```python
from build123d import *

# Parameters (mm, degrees)
CSK_FOR_M2_COUNTERSUNK_FLAT_HEAD_SCREW1_D           = 2.2
CSK_FOR_M2_COUNTERSUNK_FLAT_HEAD_SCREW1_CSINK_D     = 4.4
CSK_FOR_M2_COUNTERSUNK_FLAT_HEAD_SCREW1_CSINK_ANGLE = 90
CUT_EXTRUDE1_DEPTH                                  = 9.319
CUT_EXTRUDE1_DEPTH_BACK                             = 1.3
FILLET1_R                                           = 3
FILLET2_R                                           = 2
CUT_EXTRUDE3_START                                  = -1.35
CUT_EXTRUDE3_DEPTH                                  = 1.35
M4_TAPPED_HOLE2_D                                   = 3.3
M4_TAPPED_HOLE2_DEPTH                               = 10.1
M4_TAPPED_HOLE2_TIP                                 = 0.991420021
M2_5_TAPPED_HOLE1_D                                 = 2.05
M2_5_TAPPED_HOLE1_DEPTH                             = 6.35
M2_5_TAPPED_HOLE1_TIP                               = 0.615882135
CUT_EXTRUDE4_REACH                                  = 51.335
SKETCH11_OUTSIDE_W                                  = 62.978
SKETCH11_OUTSIDE_H                                  = 62.978
CUT_EXTRUDE2_DEPTH                                  = 50.335229157
FILLET3_R                                           = 1
CHAMFER1_SIZE                                       = 1
M4_TAPPED_HOLE1_AT_2_COUNT                          = 2
M4_TAPPED_HOLE1_AT_2_PITCH                          = 22
FILLET4_R                                           = 0.5


with BuildPart() as part:
    # Sketch1 → Revolve1 (revolve)
    with BuildSketch(Plane(origin=(0, 0, 0), x_dir=(0, 0, -1), z_dir=(1, 0, 0))):
        Polygon((13.2, 3.5), (13.2, 18.844), (15, 18.844), (15, 37.094), (23, 37.094), (23, 16.013248777), (23, 0), (8.5, 0), (5.5, 0), (5.5, 1.35), (3.75, 1.35), (3.75, 3.5), align=None)
    revolve(axis=Axis((0, 0, 0), (0, 1, 0)))

    # CSK for M2 Countersunk Flat Head Screw1 (through all)
    with Locations(Plane(origin=(0, 3.5, 0), x_dir=(1, 0, 0), z_dir=(0, 1, 0))):
        with Locations((0, 6.5), (-5.629165125, -3.25), (5.629165125, -3.25)):
            CounterSinkHole(CSK_FOR_M2_COUNTERSUNK_FLAT_HEAD_SCREW1_D / 2, CSK_FOR_M2_COUNTERSUNK_FLAT_HEAD_SCREW1_CSINK_D / 2, counter_sink_angle=CSK_FOR_M2_COUNTERSUNK_FLAT_HEAD_SCREW1_CSINK_ANGLE)

    # Sketch5 → Cut-Extrude1 (cut, two sides: drawn at the far end of the back side and taken through both)
    with BuildSketch(Plane(origin=(0, 3.5, 0), x_dir=(1, 0, 0), z_dir=(0, 1, 0)).offset(-CUT_EXTRUDE1_DEPTH_BACK)):
        with BuildLine():
            Line((-13.5, -18.62122445), (-13.5, -29.562959847))
            Line((-13.5, -29.562959847), (13.5, -29.562959847))
            Line((13.5, -29.562959847), (13.5, -18.62122445))
            ThreePointArc((13.5, -18.62122445), (16.584015432, -15.936449797), (19.14388926, -12.748))
            Line((19.14388926, -12.748), (13.93421226, -12.748))
            Line((13.93421226, -12.748), (7.5, -6.748))
            Line((7.5, -6.748), (-7.5, -6.748))
            Line((-7.5, -6.748), (-13.93421226, -12.748))
            Line((-13.93421226, -12.748), (-19.14388926, -12.748))
            ThreePointArc((-19.14388926, -12.748), (-16.584015432, -15.936449797), (-13.5, -18.62122445))
        make_face()
    extrude(amount=CUT_EXTRUDE1_DEPTH + CUT_EXTRUDE1_DEPTH_BACK, mode=Mode.SUBTRACT)

    # Fillet1
    fillet1_edges = [part.edges().sort_by_distance(p)[0] for p in [
        (-19.14388926, 7.5095, 12.748),
        (-13.93421226, 7.5095, 12.748),
        (13.93421226, 7.5095, 12.748),
        (19.14388926, 7.5095, 12.748),
    ]]
    fillet(fillet1_edges, radius=FILLET1_R)

    # Fillet2
    fillet2_edges = [part.edges().sort_by_distance(p)[0] for p in [
        (12.06906123, 3.5, -5.345817152),
    ]]
    fillet(fillet2_edges, radius=FILLET2_R)

    # Sketch14 → Cut-Extrude3 (cut)
    with BuildSketch(Plane.XZ.offset(CUT_EXTRUDE3_START)):
        with BuildLine():
            Line((1.1, -6.5), (1.1, -5.388877434))
            ThreePointArc((1.1, -5.388877434), (4.763139721, -2.75), (5.216904756, 1.741810773))
            Line((5.216904756, 1.741810773), (6.179165125, 2.297372056))
            ThreePointArc((6.179165125, 2.297372056), (6.581793069, 3.8), (5.079165125, 4.202627944))
            Line((5.079165125, 4.202627944), (4.116904756, 3.647066661))
            ThreePointArc((4.116904756, 3.647066661), (0, 5.5), (-4.116904756, 3.647066661))
            Line((-4.116904756, 3.647066661), (-5.079165125, 4.202627944))
            ThreePointArc((-5.079165125, 4.202627944), (-6.581793069, 3.8), (-6.179165125, 2.297372056))
            Line((-6.179165125, 2.297372056), (-5.216904756, 1.741810773))
            ThreePointArc((-5.216904756, 1.741810773), (-4.763139721, -2.75), (-1.1, -5.388877434))
            Line((-1.1, -5.388877434), (-1.1, -6.5))
            ThreePointArc((-1.1, -6.5), (0, -7.6), (1.1, -6.5))
        make_face()
    extrude(amount=CUT_EXTRUDE3_DEPTH, mode=Mode.SUBTRACT)

    # M4 Tapped Hole2
    with Locations(Plane(origin=(0, 37.094, 0), x_dir=(-1, 0, 0), z_dir=(0, 1, 0))):
        with Locations((16.454482672, 9.5), (0, -19), (-16.454482672, 9.5)):
            Hole(M4_TAPPED_HOLE2_D / 2, depth=M4_TAPPED_HOLE2_DEPTH)
            with Locations((0, 0, -(M4_TAPPED_HOLE2_DEPTH + M4_TAPPED_HOLE2_TIP / 2))):  # 118° drill point
                Cone(0, M4_TAPPED_HOLE2_D / 2, M4_TAPPED_HOLE2_TIP, mode=Mode.SUBTRACT)

    # M2.5 Tapped Hole1
    with Locations(Plane(origin=(0, 12.819, 0), x_dir=(-1, 0, 0), z_dir=(0, -1, 0))):
        with Locations((-10.4775, -15.748), (10.4775, -15.748)):
            Hole(M2_5_TAPPED_HOLE1_D / 2, depth=M2_5_TAPPED_HOLE1_DEPTH)
            with Locations((0, 0, -(M2_5_TAPPED_HOLE1_DEPTH + M2_5_TAPPED_HOLE1_TIP / 2))):  # 118° drill point
                Cone(0, M2_5_TAPPED_HOLE1_D / 2, M2_5_TAPPED_HOLE1_TIP, mode=Mode.SUBTRACT)

    # Sketch15 → Cut-Extrude4 (cut, up to next)
    with BuildSketch(Plane.XZ, mode=Mode.PRIVATE) as cut_extrude4_sk1:
        with BuildLine():
            Line((15.115943687, 12.748), (17.463576266, 12.748))
            ThreePointArc((17.463576266, 12.748), (18.982358673, 12.335141279), (20.083112706, 11.2102))
            ThreePointArc((20.083112706, 11.2102), (0, 23), (-20.083112706, 11.2102))
            ThreePointArc((-20.083112706, 11.2102), (-18.982358673, 12.335141279), (-17.463576266, 12.748))
            Line((-17.463576266, 12.748), (-15.115943687, 12.748))
            Line((-15.115943687, 12.748), (15.115943687, 12.748))
        make_face()
    cut_extrude4_tool1 = extrude(cut_extrude4_sk1.sketch, amount=-CUT_EXTRUDE4_REACH, mode=Mode.PRIVATE) & part.part
    add(cut_extrude4_tool1.solids().sort_by_distance((0, 0, 16.923735))[0], mode=Mode.SUBTRACT)

    # Sketch11 outside → Cut-Extrude2 (cut, through all)
    with BuildSketch(Plane(origin=(0, 0, 0), x_dir=(1, 0, 0), z_dir=(0, 1, 0))):
        Rectangle(SKETCH11_OUTSIDE_W, SKETCH11_OUTSIDE_H)
        with BuildLine():
            Line((13.983717047, 18.260768263), (20.411593144, 10.600323832))
            ThreePointArc((20.411593144, 10.600323832), (0, -23), (-20.411593144, 10.600323832))
            Line((-20.411593144, 10.600323832), (-13.983717047, 18.260768263))
            ThreePointArc((-13.983717047, 18.260768263), (0, 23), (13.983717047, 18.260768263))
        make_face(mode=Mode.SUBTRACT)
    extrude(amount=CUT_EXTRUDE2_DEPTH, mode=Mode.SUBTRACT)

    # Fillet3
    # the kernel refuses this fillet: 1 mm, written as the material it takes off along each edge
    with BuildSketch(Plane(origin=(0, 0, 0), x_dir=(-0.8322161318186808, 0, -0.5544513594002202), z_dir=(0.5544513594002202, 0, -0.8322161318186808))) as fillet3_piece_1:
        with BuildLine():
            CenterArc((23 - FILLET3_R, FILLET3_R), FILLET3_R, 270, 90)
            Line((23 - FILLET3_R, 0), (23, 0))
            Line((23, 0), (23, FILLET3_R))
        make_face()
    revolve(axis=Axis((0, 0, 0), (0, 1, 0)), revolution_arc=62.84276799, mode=Mode.SUBTRACT)
    with BuildSketch(Plane(origin=(17.463576266, 0, 9.748), x_dir=(0, 0, 1), z_dir=(-1, 0, 0))) as fillet3_piece_2:
        with BuildLine():
            CenterArc((3 - FILLET3_R, FILLET3_R), FILLET3_R, 270, 90)
            Line((3, FILLET3_R), (3, 0))
            Line((3, 0), (3 - FILLET3_R, 0))
        make_face()
    revolve(axis=Axis((17.463576266, 0, 9.748), (0, 1, 0)), revolution_arc=60.830166101, mode=Mode.SUBTRACT)
    with BuildSketch(Plane(origin=(-17.463576266, 0, 9.748), x_dir=(-0.8731788133022929, 0, 0.48739999999999956), z_dir=(-0.48739999999999956, 0, -0.8731788133022929))) as fillet3_piece_3:
        with BuildLine():
            CenterArc((3 - FILLET3_R, FILLET3_R), FILLET3_R, 270, 90)
            Line((3 - FILLET3_R, 0), (3, 0))
            Line((3, 0), (3, FILLET3_R))
        make_face()
    revolve(axis=Axis((-17.463576266, 0, 9.748), (0, 1, 0)), revolution_arc=60.830166101, mode=Mode.SUBTRACT)
    with BuildSketch(Plane(origin=(17.463576266, 0, 12.748), x_dir=(0, 1, 0), z_dir=(-1, 0, 0))) as fillet3_piece_4:
        with BuildLine():
            CenterArc((FILLET3_R, FILLET3_R), FILLET3_R, 180, 90)
            Line((0, FILLET3_R), (0, 0))
            Line((0, 0), (FILLET3_R, 0))
        make_face()
    extrude(amount=34.927152532, mode=Mode.SUBTRACT)
    with BuildSketch(Plane(origin=(0, 37.094, 0), x_dir=(-0.8320605059369173, 0, -0.5546848785211302), z_dir=(0.5546848785211302, 0, -0.8320605059369173))) as fillet3_piece_5:
        with BuildLine():
            CenterArc((23 - FILLET3_R, -FILLET3_R), FILLET3_R, 0, 90)
            Line((23 - FILLET3_R, 0), (23, 0))
            Line((23, 0), (23, -FILLET3_R))
        make_face()
    revolve(axis=Axis((0, 37.094, 0), (0, 1, 0)), revolution_arc=247.378025481, mode=Mode.SUBTRACT)
    with BuildSketch(Plane(origin=(0, 37.094, 0), x_dir=(0.6905501820120585, 0, -0.7232844849180111), z_dir=(0.7232844849180111, 0, 0.6905501820120585))) as fillet3_piece_6:
        with BuildLine():
            CenterArc((23 - FILLET3_R, -FILLET3_R), FILLET3_R, 0, 90)
            Line((23 - FILLET3_R, 0), (23, 0))
            Line((23, 0), (23, -FILLET3_R))
        make_face()
    revolve(axis=Axis((0, 37.094, 0), (0, 1, 0)), revolution_arc=87.347352667, mode=Mode.SUBTRACT)
    with BuildSketch(Plane(origin=(0, 0, 0), x_dir=(-0.6905501820120575, 0, -0.7232844849180122), z_dir=(-0.7232844849180122, 0, 0.6905501820120575))) as fillet3_piece_7:
        with BuildLine():
            CenterArc((23 - FILLET3_R, -FILLET3_R), FILLET3_R, 0, 90)
            Line((23 - FILLET3_R, 0), (23, 0))
            Line((23, 0), (23, -FILLET3_R))
        make_face()
    revolve(axis=Axis((0, 0, 0), (0, -1, 0)), revolution_arc=87.347352667, mode=Mode.SUBTRACT)
    with BuildSketch(Plane(origin=(0, 0, 0), x_dir=(0.8731788133022923, 0, 0.48740000000000056), z_dir=(-0.48740000000000056, 0, 0.8731788133022923))) as fillet3_piece_8:
        with BuildLine():
            CenterArc((23 - FILLET3_R, FILLET3_R), FILLET3_R, 270, 90)
            Line((23 - FILLET3_R, 0), (23, 0))
            Line((23, 0), (23, FILLET3_R))
        make_face()
    revolve(axis=Axis((0, 0, 0), (0, 1, 0)), revolution_arc=62.84276799, mode=Mode.SUBTRACT)
    with BuildSketch(Plane(origin=(-22.018562168, 37.094, -8.685212724), x_dir=(0, -1, 0), z_dir=(0.6427876096865434, 0, -0.7660444431189748))) as fillet3_piece_9:
        with BuildLine():
            CenterArc((FILLET3_R, -FILLET3_R), FILLET3_R, 90, 90)
            Line((0, -FILLET3_R), (0, 0))
            Line((0, 0), (FILLET3_R, 0))
        make_face()
    extrude(amount=15, mode=Mode.SUBTRACT)
    with BuildSketch(Plane(origin=(12.376748023, 37.094, -20.175879371), x_dir=(-0.7660444431189747, 0, 0.6427876096865432), z_dir=(0.6427876096865434, 0, 0.7660444431189748)), Plane(origin=(12.376748023, 0, -20.175879371), x_dir=(0, 1, 0), z_dir=(0.6427876096865434, 0, 0.7660444431189748)), Plane(origin=(-22.018562168, 0, -8.685212724), x_dir=(0, 1, 0), z_dir=(0.6427876096865434, 0, -0.7660444431189748))) as fillet3_piece_10:
        with BuildLine():
            CenterArc((FILLET3_R, FILLET3_R), FILLET3_R, 180, 90)
            Line((0, FILLET3_R), (0, 0))
            Line((0, 0), (FILLET3_R, 0))
        make_face()
    extrude(amount=15, mode=Mode.SUBTRACT)

    # Chamfer1
    chamfer1_edges = [part.edges().sort_by_distance(p)[0] for p in [
        (0, 37.094, 15),
    ]]
    chamfer(chamfer1_edges, length=CHAMFER1_SIZE)

    # Sketch12 → M4 Tapped Hole1 (revolve, cut)
    with BuildSketch(Plane(origin=(17.197655095, 10.094, -14.430546047), x_dir=(-0.6427876096865435, 0, -0.7660444431189747), z_dir=(0, 1, 0))):
        Polygon((0, 0), (0, 11.091420021), (1.65, 10.1), (1.65, 0), align=None)
    m4_tapped_hole1 = revolve(axis=Axis((22.062037309, 10.094, -18.512247369), (-0.7660444431189746, 0, 0.6427876096865435)), mode=Mode.SUBTRACT)

    # M4 Tapped Hole1 at 2: M4 Tapped Hole1 ×2
    with Locations(*[(0, i * M4_TAPPED_HOLE1_AT_2_PITCH, 0) for i in range(1, M4_TAPPED_HOLE1_AT_2_COUNT)]):
        add(m4_tapped_hole1, mode=Mode.SUBTRACT)

    # Mirror1: M4 Tapped Hole1 across plane
    add(m4_tapped_hole1.mirror(Plane(origin=(0, 0, 0), x_dir=(0, 0, 1), z_dir=(1, 0, 0))), mode=Mode.SUBTRACT)

    # Mirror1 copy 1 sketch → Mirror1 copy 1 (revolve, cut)
    with BuildSketch(Plane(origin=(-17.197655095, 32.094, -14.430546047), x_dir=(0.6427876096865435, 0, -0.7660444431189747), z_dir=(0, 1, 0))):
        Polygon((0, 0), (0, -11.091420021), (1.65, -10.1), (1.65, 0), align=None)
    revolve(axis=Axis((-22.062037309, 32.094, -18.512247369), (-0.7660444431189746, 0, -0.6427876096865435)), mode=Mode.SUBTRACT)

    # Fillet4
    fillet4_edges = [part.edges().sort_by_distance(p)[0] for p in [
        (-7.5, 2.85, 6.748),
        (7.5, 2.85, 6.748),
    ]]
    fillet(fillet4_edges, radius=FILLET4_R)


solid = part.part
```
Design review of the part built by this model. Coordinates are the model's own, in mm. A direction names the side the tool comes from. Coordinates: 2 decimals unless noted, no trailing zeros. Loops run counter-clockwise (first coordinate to the right, second up) from the corner with the lowest first, then second, coordinate; pieces in that order, holes last. Notation, with made-up numbers: (37.25, -5.5) - (65.25, -5.5) arc R31 ccw to (65.25, 30.5) - close; hole circle Ø2 at (57, 64.5). An arc over 180 degrees is marked (long way). Use CSV: the item, a comma, the result in double quotes. Start each with the question number.
1) Wall thickness on L1, parallel to Z at x = 0, y = 28.25; L2, parallel to Z at x = -0.5, y = 26; L3, parallel to Y at x = 1.5, z = -5: over which ranges is each line inside the solid? List them lowest first. Write a range as from..to.
2) For pin 1 Ø1 at (y, z) = (15.5, -16.5) entering from +X; pin 2 Ø3 at (x, y) = (5, 6) entering from -Z; pin 3 Ø2 at (x, z) = (9.5, -2.5) entering from +Y, all flat-tipped, find the tip position at first contact; note any pin that passes through.
3) Consider section C-C on y = 15.5. Give the number of separate pieces and of enclosed holes in the cut face, then the cut area to 3 significant figures.
4) Consider section D-D on y = 28. Write out the cut boundary in (x, z).
5) The part is to be moulded in two halves that separate along X. For faces 5 (the cylindrical face through (-17.024, 36.793, -14.194)), 6 (the cylindrical face through (-6.645, 1.45, 3.671)), 7 (the cylindrical face through (16.934, 36.793, -14.301)), 8 (the conical face through (0.037, 26.175, -18.716)), say which applies: +X half, -X half, draft (parallel to the pull), parting line (faces both ways), or undercut.
6) Consider section B-B on y = 22.5. Write out the cut boundary in (x, z), then the cut area to 3 significant figures.
7) Consider section A-A on z = 0. Write out the cut boundary in (x, y), then the cut area to 3 significant figures.
8) Tool access review of faces 1 (the flat face through (0, 2, 12.748)), 2 (the flat face through (-11.525, 7.435, 10.501)), 3 (the flat face through (1, 1.35, 4)), 4 (the cylindrical face through (17.98, 31.97, 8.87)): name each direction out of +Z, -Z, +X, -X, +Y, -Y from which nothing blocks a thin tool from reaching the whole face with its end or side.
Geometry says:
1,L1,"-23..-20.65, -17.35..-15, 15..23"
1,L2,"-22.99..-14.99, 14.99..22.99"
1,L3,"1.35..3.42"
2,pin 1,"x = 15.88"
2,pin 2,"z = -22.73"
2,pin 3,"y = 3.5"
3,separate pieces,"1"
3,enclosed holes,"3"
3,area,"1,100 mm^2"
4,outline,"(-20.41, -10.6) - (-13.98, -18.26) arc R23 ccw to (13.98, -18.26) - (20.41, -10.6) arc R23 ccw (long way) to start; hole circle Ø3.3 at (-16.45, 9.5); hole circle Ø30 at (0, 0); hole circle Ø3.3 at (0, -19); hole circle Ø3.3 at (16.45, 9.5)"
5,face 5,"-X half"
5,face 6,"undercut"
5,face 7,"+X half"
5,face 8,"undercut"
6,outline,"(-20.41, -10.6) - (-13.98, -18.26) arc R23 ccw to (13.98, -18.26) - (20.41, -10.6) arc R23 ccw (long way) to start; hole circle Ø30 at (0, 0)"
6,area,"948 mm^2"
7,outline,"(-23, 1) arc R1 ccw to (-22, 0) - (-5.5, 0) - (-5.5, 1.35) - (-3.75, 1.35) - (-3.75, 3.5) - (-11.2, 3.5) arc R2 cw to (-13.2, 5.5) - (-13.2, 18.84) - (-15, 18.84) - (-15, 36.09) - (-16, 37.09) - (-22, 37.09) arc R1 ccw to (-23, 36.09) - close; (3.75, 1.35) - (5.5, 1.35) - (5.5, 0) - (22, 0) arc R1 ccw to (23, 1) - (23, 36.09) arc R1 ccw to (22, 37.09) - (16, 37.09) - (15, 36.09) - (15, 18.84) - (13.2, 18.84) - (13.2, 5.5) arc R2 cw to (11.2, 3.5) - (3.75, 3.5) - close"
7,area,"723 mm^2"
8,face 1,"+Z, +X, -X, -Y"
8,face 2,"+Z"
8,face 3,"-Y"
8,face 4,"+Y"
